Design review of the part built by this model. Coordinates are the model's own, in mm. Coordinates: 2 decimals unless noted, no trailing zeros. Loops run counter-clockwise (first coordinate to the right, second up) from the corner with the lowest first, then second, coordinate; pieces in that order, holes last. Notation, with made-up numbers: (48.5, -19) - (85.5, -19) arc R11 cw to (85.5, -6) - close; hole circle Ø9 at (71, -10). An arc over 180 degrees is marked (long way). One line per question, with ' | ' between items.
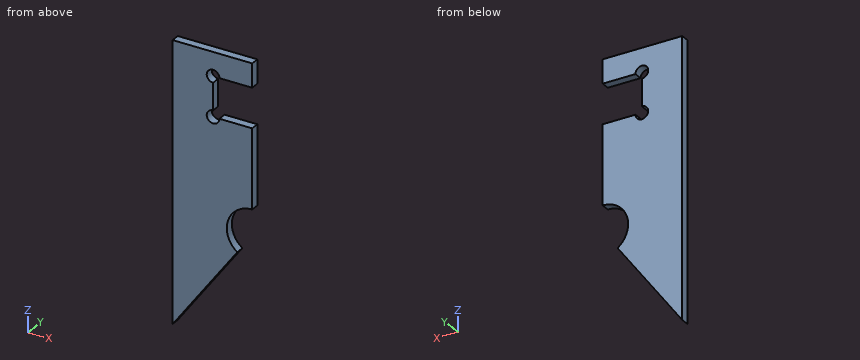
Autodesk Inventor part; units mm, degrees
ref_plane "YZ Plane" through (0, 0, 0) normal (1, 0, 0) x (0, 1, 0)
ref_plane "XZ Plane" through (0, 0, 0) normal (0, 1, 0) x (-1, 0, 0)
ref_plane "XY Plane" through (0, 0, 0) normal (0, 0, 1) x (1, 0, 0)
sketch "スケッチ1" plane through (0, 0, 0) normal (0, 1, 0) x (-1, 0, 0)
  line L0 (0, 0) -> (25, 0)
  line L1 (25, 0) -> (25, -33)
  line L2 (25, -33) -> (0, -33)
  line L3 (0, -33) -> (0, 0)
  line L4 (0, -33) -> (25, -27)
  line L5 (0, -33) -> (25, -67.4095)
  line L6 (25, -67.4095) -> (25, -33)
  dimension "d0" = 25
  dimension "d1" = 33
  dimension "d2" = 27
  dimension "d3" = 36
extrude "押し出し1" add sketch "スケッチ1" along normal blind 2.65
sketch "スケッチ2" plane through (0, 2.65, 0) normal (0, 1, 0) x (1, 0, 0)
  line L0 (0, 33) -> (-25, 67.4095)
  line L1 (0, 0) -> (0, 33)
  arc A0 (-4.7023, 39.4721) -> (0, 25) centre (0, 33) ccw
  dimension "d6" = 8
extrude "押し出し2" cut sketch "スケッチ2" against normal blind 2.65
sketch "スケッチ3" plane through (0, 2.65, 0) normal (0, 1, 0) x (1, 0, 0)
  line L0 (-25, 67.4095) -> (-25, 0)
  line L1 (-25, 0) -> (-12.3, 0)
  line L2 (-12.3, 0) -> (-12.3, -20)
  line L3 (-12.3, -20) -> (-25, -20)
  line L4 (-25, -20) -> (-25, 0)
  line L5 (0, 0) -> (0, 25)
  dimension "d9" = 20
  dimension "d10" = 12.3
extrude "押し出し3" add sketch "スケッチ3" against normal blind 2.65
sketch "スケッチ4" plane through (0, 2.65, 0) normal (0, 1, 0) x (1, 0, 0)
  line L0 (-12.3, 0) -> (0, 0)
  circle A0 centre (-12.3, 0) radius 2
  dimension "d13" = 4
extrude "押し出し4" cut sketch "スケッチ4" against normal blind 2.65
sketch "スケッチ5" plane through (0, 2.65, 0) normal (0, 1, 0) x (1, 0, 0)
  line L0 (-12.3, -2) -> (-12.3, -20)
  line L1 (-12.3, -20) -> (0, -20)
  line L2 (0, -20) -> (0, -12.5)
  line L3 (0, -12.5) -> (-12.3, -12.5)
  line L4 (-12.3, -12.5) -> (-12.3, -20)
  line L5 (-10.3, 0) -> (0, 0)
  dimension "d16" = 12.3
  dimension "d18" = 12.5
extrude "押し出し5" add sketch "スケッチ5" against normal blind 2.65
sketch "スケッチ6" plane through (0, 2.65, 0) normal (0, 1, 0) x (1, 0, 0)
  line L0 (-12.3, -12.5) -> (0, -12.5)
  point P0 (0, 0)
hole "穴1" at (-12.3, 2.65, 12.5) direction (0, -1, 0) diameter 4 end through all
properties part number "bendpart_36deg"
Q1. Take a section at A-A (x = -11.25). Give the boundary of the cut face in (y, z), plus the area to 3 significant figures.
Returned:
outline: (0, -48.48) - (2.65, -48.48) - (2.65, -1.7) - (0, -1.7) - close; (0, 14.2) - (2.65, 14.2) - (2.65, 20) - (0, 20) - close | area: 139 mm²
Q2. Take a section at D-D (x = -19.75). Give the boundary of the cut face in (y, z), plus the area to 3 significant figures.
Returned:
outline: (0, -60.18) - (2.65, -60.18) - (2.65, 20) - (0, 20) - close | area: 212 mm²
Q3. Take a section at B-B (y = 0.85). Give the boundary of the cut face in (x, z), plus the area to 3 significant figures.
Returned:
outline: (-25, -67.41) - (-4.7, -39.47) arc R8 cw to (0, -25) - (0, 0) - (-10.3, 0) arc R2 cw (long way) to (-12.3, 2) - (-12.3, 10.5) arc R2 cw (long way) to (-10.3, 12.5) - (0, 12.5) - (0, 20) - (-25, 20) - close | area: 1,500 mm²
Q4. Take a section at C-C (z = 3.5). Give the boundary of the cut face in (x, y).
Returned:
outline: (-25, 0) - (-12.3, 0) - (-12.3, 2.65) - (-25, 2.65) - close
Q5. To check wall thickness, follow line 1 along Z through (x, y) = (-14, 2.15); line 2 along Z through (x, y) = (-11.5, 1.75); line 3 along X through (y, z) = (2, -37.5). State the ranges of each line that lie inside material, in increasing order.
Returned:
line 1: z = -52.27 to -1.05, 1.05 to 11.45, 13.55 to 20 | line 2: z = -48.83 to -1.83, 14.33 to 20 | line 3: x = -25 to -6.61
Q6. For pin 1 (0.8 mm diameter, centred on x = -4.5, y = 1, fed in from -Z); pin 2 (1 mm diameter, centred on x = -3.5, z = -41.5, fed in from -Y), all flat-tipped, find the tip position at first contact; note any pin that passes through.
Returned:
pin 1: stops at z = -39.74 | pin 2: passes through
